The model under review builds one solid part; all positions refer to its coordinate system, in mm. A direction names the side the tool comes from. Give positions to 0.01 mm unless a question says otherwise; leave off trailing zeros. Loops run counter-clockwise (first coordinate to the right, second up) from the corner with the lowest first, then second, coordinate; pieces in that order, holes last. Notation, with made-up numbers: (-11.75, 27.25) -> (37.25, 27.25) arc R30 ccw to (37.25, 65.25) -> close; hole circle Ø9 at (87.25, 26). An arc over 180 degrees is marked (long way). Write each question's results on one line, items separated by ' | '. Start each with the question number.
Q1. We need section B-B (x = 5.25). Write out the cut boundary in (y, z), plus the area to 3 significant figures.
Q2. We need section A-A (z = 14). Write out the cut boundary in (x, y), plus the area to 3 significant figures.
Q3. Insertion check: pin 1 Ø2 at (x, y) = (6, 109.5) entering from +Z; pin 2 Ø2 at (x, y) = (6, 103.5) entering from -Z; pin 3 Ø3 at (x, z) = (4, -39) entering from -Y. Each pin has a flat end and moves straight along its axis. Give the tip position at first contact, or say it passes through.
Q4. We need section C-C (y = 36). Write out the cut boundary in (x, z), plus the area to 3 significant figures.
Q5. Wall thickness on L1, parallel to Z at x = 1.5, y = 23.5; L2, parallel to Z at x = 1.25, y = 49.5; L3, parallel to Z at x = 5.25, y = 122.5: over which ranges is each line inside the solid? List them lowest first. Write a range as [from, to].
Q6. Machinability: for faces 1 (the face through (3.882, 43.828, 11.744)), 2 (the face through (0, 73, 21)), which of the approach directions +Z, -Z, +X, -X, +Y, -Y give a long, thin tool a straight path to every point of the face, cutting with its end or side? Answer none if there is none.
Q7. We need section D-D (y = 117.5). Write out the cut boundary in (x, z).
from build123d import *

# Parameters (mm, degrees)
F1_DEPTH = 7.874
F2_R     = 21.289722
F3_R     = 5.08


with BuildPart() as f1:
    # F0 (on Right) → F1 (new body)
    with BuildSketch(Plane.YZ):
        Polygon((0, 25.4), (0, 0), (88.9, 23.820683), (120.941612, 32.406207), (171.741612, 46.018026), (171.741612, 71.418026), align=None)
        Polygon((120.941612, 32.406207), (88.9, 23.820683), (0, -50.775274), (0, -69.075855), align=None)
    extrude(amount=F1_DEPTH)

    # F2
    f2_edges = [f1.edges().sort_by_distance(p)[0] for p in [
        (3.937, 171.741612, 46.018026),
    ]]
    fillet(f2_edges, radius=F2_R)

    # F3
    f3_edges = [f1.edges().sort_by_distance(p)[0] for p in [
        (3.937, 171.741612, 71.418026),
    ]]
    fillet(f3_edges, radius=F3_R)


solid = f1.part
Output:
1) outline: (0, -69.08) -> (120.94, 32.41) -> (155.96, 41.79) arc R21.29 ccw to (171.74, 62.35) -> (171.74, 64.8) arc R5.08 ccw to (165.35, 69.7) -> (0, 25.4) -> (0, 0) -> (88.9, 23.82) -> (0, -50.78) -> close | area: 6,220 mm2
2) outline: (0, 0) -> (7.87, 0) -> (7.87, 52.25) -> (0, 52.25) -> close; (0, 77.2) -> (7.87, 77.2) -> (7.87, 99.01) -> (0, 99.01) -> close | area: 583 mm2
3) pin 1: z = 55.01 | pin 2: z = 16.93 | pin 3: y = 12.25
4) outline: (0, -38.87) -> (7.87, -38.87) -> (7.87, -20.57) -> (0, -20.57) -> close; (0, 9.65) -> (7.87, 9.65) -> (7.87, 35.05) -> (0, 35.05) -> close | area: 344 mm2
5) L1: [-49.36, -31.06], [6.3, 31.7] | L2: [-27.54, -9.24], [13.26, 38.66] | L3: [32.82, 58.22]
6) face 1: +X, -X | face 2: +Z, -Z, -X, +Y, -Y
7) outline: (0, 29.52) -> (7.87, 29.52) -> (7.87, 56.88) -> (0, 56.88) -> close
